Part model, mm, in its own coordinate system. A direction names the side the tool comes from. Round coordinates to 2 decimals unless told otherwise and drop trailing zeros. Loops run counter-clockwise (first coordinate to the right, second up) from the corner with the lowest first, then second, coordinate; pieces in that order, holes last. Notation, with made-up numbers: (-4.5, 59.5) - (43.5, 59.5) arc R24 ccw to (43.5, 88.5) - close; hole circle Ø5 at (-10, 21.5). An arc over 180 degrees is marked (long way). Put each result on its own line as item: value.
from build123d import *

# Parameters (mm, degrees)
EXTRUDE_1_DEPTH          = 10
SKETCH_2_W               = 231
SKETCH_2_H               = 139
EXTRUDE_1_2_DEPTH        = 3
FILLET_1_R               = 1
CHAMFER_1_SIZE           = 1
CUT_EXTRUDE_1_DEPTH      = 287.389594783
CUT_EXTRUDE_1_DEPTH_BACK = 2
SKETCH_3_W               = 71.087717772
SKETCH_3_H               = 10
SKETCH_4_W               = 21.591384664
SKETCH_4_H               = 17.851519678
SKETCH_4_W_2             = 20.271944057
SKETCH_4_H_2             = 16.15289462
SKETCH_4_W_3             = 20.32571751
SKETCH_4_H_3             = 19.635596567
SKETCH_4_W_4             = 22.15685921
SKETCH_4_H_4             = 28.871680817
CUT_EXTRUDE_2_DEPTH      = 10


with BuildPart() as part:
    # 草图1 → Extrude 1 (new body)
    with BuildSketch(Plane(origin=(0, 0, 0), x_dir=(1, 0, 0), z_dir=(0, 1, 0))):
        with BuildLine():
            Line((-117.5, 147), (117.5, 147))
            ThreePointArc((117.5, 147), (118.914213562, 146.414213562), (119.5, 145))
            Line((119.5, 145), (119.5, 2))
            ThreePointArc((119.5, 2), (118.914213562, 0.585786438), (117.5, 0))
            Line((117.5, 0), (-117.5, 0))
            ThreePointArc((-117.5, 0), (-118.914213562, 0.585786438), (-119.5, 2))
            Line((-119.5, 2), (-119.5, 145))
            ThreePointArc((-119.5, 145), (-118.914213562, 146.414213562), (-117.5, 147))
        make_face()
        with BuildLine():
            Line((-117.5, 146.4), (117.5, 146.4))
            ThreePointArc((117.5, 146.4), (118.489949494, 145.989949494), (118.9, 145))
            Line((118.9, 145), (118.9, 2))
            ThreePointArc((118.9, 2), (118.489949494, 1.010050506), (117.5, 0.6))
            Line((117.5, 0.6), (-117.5, 0.6))
            ThreePointArc((-117.5, 0.6), (-118.489949494, 1.010050506), (-118.9, 2))
            Line((-118.9, 2), (-118.9, 145))
            ThreePointArc((-118.9, 145), (-118.489949494, 145.989949494), (-117.5, 146.4))
        make_face(mode=Mode.SUBTRACT)
    extrude(amount=EXTRUDE_1_DEPTH)

    # 草图2 → Extrude 1 2 (add)
    with BuildSketch(Plane(origin=(0, 10, 0), x_dir=(1, 0, 0), z_dir=(0, 1, 0))):
        with BuildLine():
            Line((123.5, 2), (123.5, 145))
            ThreePointArc((123.5, 145), (121.742640687, 149.242640687), (117.5, 151))
            Line((117.5, 151), (-117.5, 151))
            ThreePointArc((-117.5, 151), (-121.742640687, 149.242640687), (-123.5, 145))
            Line((-123.5, 145), (-123.5, 2))
            ThreePointArc((-123.5, 2), (-121.742640687, -2.242640687), (-117.5, -4))
            Line((-117.5, -4), (117.5, -4))
            ThreePointArc((117.5, -4), (121.742640687, -2.242640687), (123.5, 2))
        make_face()
        with Locations((0, 73.5)):
            Rectangle(SKETCH_2_W, SKETCH_2_H, mode=Mode.SUBTRACT)
    extrude(amount=EXTRUDE_1_2_DEPTH)

    # 圆角1
    fillet_1_edges = [part.edges().sort_by_distance(p)[0] for p in [
        (-115.5, 11.5, -4),
        (115.5, 11.5, -4),
        (115.5, 11.5, -143),
        (-115.5, 11.5, -143),
    ]]
    fillet(fillet_1_edges, radius=FILLET_1_R)

    # 倒角1
    chamfer_1_edges = [part.edges().sort_by_distance(p)[0] for p in [
        (121.742640687, 13, -149.242640687),
        (0, 13, -151),
        (-121.742640687, 13, -149.242640687),
        (-123.5, 13, -73.5),
        (-121.742640687, 13, 2.242640687),
        (0, 13, 4),
        (121.742640687, 13, 2.242640687),
        (123.5, 13, -73.5),
    ]]
    chamfer(chamfer_1_edges, length=CHAMFER_1_SIZE)

    # 草图3 → 切除-拉伸1 (cut, two sides: drawn at the far end of the back side and taken through both)
    with BuildSketch(Plane.ZY.offset(119.5).offset(-CUT_EXTRUDE_1_DEPTH_BACK)):
        with Locations((-94.14273439, 5)):
            Rectangle(SKETCH_3_W, SKETCH_3_H)
    extrude(amount=CUT_EXTRUDE_1_DEPTH + CUT_EXTRUDE_1_DEPTH_BACK, mode=Mode.SUBTRACT)

    # 草图4 → 切除-拉伸2 (cut)
    with BuildSketch(Plane.XZ):
        with Locations((-117.828855159, -2.837454771)):
            Rectangle(SKETCH_4_W, SKETCH_4_H)
        with Locations((-118.488575463, -142.547638379)):
            Rectangle(SKETCH_4_W_2, SKETCH_4_H_2)
        with Locations((115.371142154, -142.781057231)):
            Rectangle(SKETCH_4_W_3, SKETCH_4_H_3)
        with Locations((118.925594218, 2.295642768)):
            Rectangle(SKETCH_4_W_4, SKETCH_4_H_4)
    extrude(amount=-CUT_EXTRUDE_2_DEPTH, mode=Mode.SUBTRACT)


solid = part.part
1. Probe line 1 along Z through (x, y) = (-58.5, 10.75); line 2 along X through (y, z) = (11.25, -20); line 3 along Z through (x, y) = (30, 1). List the from-to ranges inside material, lowest first. Write a range as [from, to].
A:
line 1: z = [-151, -143], [-4, 4]
line 2: x = [-123.5, -115.5], [115.5, 123.5]
line 3: z = [-147, -146.4], [-0.6, 0]
2. Band-saw the part on A-A (z = -16.5). List the corners of the cut face in (x, y).
A:
outline: (-123.5, 10) - (-119.5, 10) - (-119.5, 0) - (-118.9, 0) - (-118.9, 10) - (-115.5, 10) - (-115.5, 13) - (-122.5, 13) - (-123.5, 12) - close; (115.5, 10) - (118.9, 10) - (118.9, 0) - (119.5, 0) - (119.5, 10) - (123.5, 10) - (123.5, 12) - (122.5, 13) - (115.5, 13) - close
3. Tool access for faces 1 (the flat face through (-119.5, 5, -35)), 2 (the flat face through (2, 5, -0.6)), 3 (the flat face through (-118.9, 5, -132)), 4 (the flat face through (2, 5, 0)), 5 (the flat face through (119.5, 5, -73)): list every direction of +Z, -Z, +X, -X, +Y, -Y with a clear straight run to the whole face (end or side of a thin tool).
A:
face 1: +Z, -Z, -X, -Y
face 2: +X, -X, -Y
face 3: +Z, -Z, -Y
face 4: +Z, +X, -X, -Y
face 5: +Z, -Z, +X, -Y
4. Band-saw the part on C-C (y = 2.5). List the corners of the cut face in (x, z), plus the area to 3 significant figures.
A:
outline: (-119.5, -134.47) - (-118.9, -134.47) - (-118.9, -129.69) - (-119.5, -129.69) - close; (-119.5, -58.6) - (-118.9, -58.6) - (-118.9, -11.76) - (-119.5, -11.76) - close; (-108.35, -147) - (105.21, -147) - (105.21, -146.4) - (-108.35, -146.4) - close; (-107.03, -0.6) - (107.85, -0.6) - (107.85, 0) - (-107.03, 0) - close; (118.9, -132.96) - (119.5, -132.96) - (119.5, -12.14) - (118.9, -12.14) - close
area: 361 mm²
5. Band-saw the part on B-B (x = 43). List the corners of the cut face in (y, z), plus the area to 3 significant figures.
A:
outline: (0, -147) - (10, -147) - (10, -151) - (12, -151) - (13, -150) - (13, -143) - (10, -143) - (10, -146.4) - (0, -146.4) - close; (0, -0.6) - (10, -0.6) - (10, -4) - (13, -4) - (13, 3) - (12, 4) - (10, 4) - (10, 0) - (0, 0) - close
area: 59.0 mm²
6. Pin check, flat tips, straight feed: P1, Ø1.4, axis at y = 6.5, z = -132, coming from the -X side; P2, Ø3, axis at y = 5, z = -45, coming from the +X side; P3, Ø1, axis at x = -43, y = 5, coming from the -Z side. Stop position of each tip, or through.
A:
P1: stops at x = -119.5
P2: stops at x = 119.5
P3: stops at z = -147
7. Band-saw the part on D-D (z = -68). List the corners of the cut face in (x, y), plus the area to 3 significant figures.
A:
outline: (-123.5, 10) - (-115.5, 10) - (-115.5, 13) - (-122.5, 13) - (-123.5, 12) - close; (115.5, 10) - (118.9, 10) - (118.9, 0) - (119.5, 0) - (119.5, 10) - (123.5, 10) - (123.5, 12) - (122.5, 13) - (115.5, 13) - close
area: 53.0 mm²
8. Two-plate mould, pull along X, no slides. Class faces 6 (the flat face through (-119.5, 5, -132)), 7 (the conical face through (121.196, 12.715, 1.778)), 8 (the flat face through (-118.9, 5, -35)): pulls with the +X half, pulls with the -X half, needs draft (parallel to the pull), parting line crosses it, or undercut.
A:
face 6: pulls with the -X half
face 7: pulls with the +X half
face 8: undercut
